Work out the finished part from the listing and answer in its coordinate system (mm). Face numbers are marked on the shaded views. A direction names the side the tool comes from. Give positions to 0.01 mm unless a question says otherwise; leave off trailing zeros. One line per item, written item: value.
from build123d import *

# Parameters (mm, degrees)
SKETCH1_W                   = 105
SKETCH1_H                   = 70
BOSS_EXTRUDE1_DEPTH         = 3
FILLET4_R                   = 3
FILLET5_R                   = 3
FILLET6_R                   = 3
M5X0_8_TAPPED_HOLE2_D       = 4.2
SKETCH16_6_W                = 34
SKETCH16_6_H                = 61
SKETCH16_6_W_2              = 30
SKETCH16_6_H_2              = 57
BOSS_EXTRUDE3_DEPTH         = 20
CUT_EXTRUDE8_REACH          = 129.334
SKETCH21_W                  = 30
SKETCH21_H                  = 57
SKETCH20_W                  = 34
SKETCH20_H                  = 61
BOSS_EXTRUDE4_DEPTH         = 2
SKETCH22_W                  = 34
SKETCH22_H                  = 61
CUT_EXTRUDE9_DEPTH          = 1.5
FILLET8_R                   = 3
SKETCH26_R                  = 6
CUT_EXTRUDE10_DEPTH         = 1.5
M3_TAPPED_HOLE1_D           = 2.5
M3_TAPPED_HOLE1_DEPTH       = 7.5
M3_TAPPED_HOLE1_TIP         = 0.751075774
SKETCH33_W                  = 1.5
SKETCH33_H                  = 5
CUT_EXTRUDE11_DEPTH         = 3
M3_TAPPED_HOLE2_D           = 2.5
M3_TAPPED_HOLE2_DEPTH       = 7.5
M3_TAPPED_HOLE2_TIP         = 0.751075774
M3_TAPPED_HOLE3_D           = 2.5
M3_TAPPED_HOLE3_DEPTH       = 7.5
M3_TAPPED_HOLE3_TIP         = 0.751075774
CUT_EXTRUDE12_REACH         = 101.423
SKETCH37_W                  = 10
SKETCH37_H                  = 10
SKETCH39_R                  = 3
CUT_EXTRUDE13_DEPTH         = 1.5
TAP_DRILL_FOR_M4X0_7_TAP2_D = 3.3


with BuildPart() as part:
    # Sketch1 → Boss-Extrude1 (new body)
    with BuildSketch(Plane.XY):
        with Locations((52.5, 35)):
            Rectangle(SKETCH1_W, SKETCH1_H)
    extrude(amount=BOSS_EXTRUDE1_DEPTH)

    # Fillet4
    fillet4_edges = [part.edges().sort_by_distance(p)[0] for p in [
        (105, 0, 1.5),
        (105, 70, 1.5),
    ]]
    fillet(fillet4_edges, radius=FILLET4_R)

    # Fillet5
    fillet5_edges = [part.edges().sort_by_distance(p)[0] for p in [
        (51, 70, 3),
        (105, 35, 3),
        (51, 0, 3),
        (104.121320344, 69.121320344, 3),
        (104.121320344, 0.878679656, 3),
    ]]
    fillet(fillet5_edges, radius=FILLET5_R - 0.0001)  # a hair under: the kernel refuses the full size

    # Fillet6
    fillet6_edges = [part.edges().sort_by_distance(p)[0] for p in [
        (0, 35, 3),
        (0, 0.878650367, 2.121349633),
        (0, 69.121349633, 2.121349633),
    ]]
    fillet(fillet6_edges, radius=FILLET6_R - 0.0001)  # a hair under: the kernel refuses the full size

    # M5x0.8 Tapped Hole2 (through all)
    with Locations(Plane(origin=(4, 66, 3), x_dir=(1, 0, 0), z_dir=(0, 0, 1))):
        with Locations((0, 0), (0, -62)):
            Hole(M5X0_8_TAPPED_HOLE2_D / 2)

    # Sketch16<6> → Boss-Extrude3 (add)
    with BuildSketch(Plane.XY.offset(3)):
        with Locations((83, 35)):
            Rectangle(SKETCH16_6_W, SKETCH16_6_H)
        with Locations((83, 35)):
            Rectangle(SKETCH16_6_W_2, SKETCH16_6_H_2, mode=Mode.SUBTRACT)
    extrude(amount=-BOSS_EXTRUDE3_DEPTH)

    # Sketch21 → Cut-Extrude8 (cut, up to next)
    with BuildSketch(Plane(origin=(0, 0, 0), x_dir=(-1, 0, 0), z_dir=(0, 0, -1)), mode=Mode.PRIVATE) as cut_extrude8_sk1:
        with Locations((-83, 35)):
            Rectangle(SKETCH21_W, SKETCH21_H)
    cut_extrude8_tool1 = extrude(cut_extrude8_sk1.sketch, amount=-CUT_EXTRUDE8_REACH, mode=Mode.PRIVATE) & part.part
    add(cut_extrude8_tool1.solids().sort_by_distance((83, 35, 0))[0], mode=Mode.SUBTRACT)

    # Sketch20 → Boss-Extrude4 (add)
    with BuildSketch(Plane(origin=(0, 0, -17), x_dir=(-1, 0, 0), z_dir=(0, 0, -1))):
        with Locations((-83, 35)):
            Rectangle(SKETCH20_W, SKETCH20_H)
    extrude(amount=BOSS_EXTRUDE4_DEPTH)

    # Sketch22 → Cut-Extrude9 (cut)
    with BuildSketch(Plane.XY.offset(3)):
        with Locations((83, 35)):
            Rectangle(SKETCH22_W, SKETCH22_H)
    extrude(amount=-CUT_EXTRUDE9_DEPTH, mode=Mode.SUBTRACT)

    # Fillet8
    fillet8_edges = [part.edges().sort_by_distance(p)[0] for p in [
        (100, 35, -19),
        (83, 4.5, -19),
        (66, 35, -19),
        (83, 65.5, -19),
    ]]
    fillet(fillet8_edges, radius=FILLET8_R)

    # Sketch26 → Cut-Extrude10 (cut)
    with BuildSketch(Plane.XY.offset(3)):
        with Locations((66, 35)):
            Circle(SKETCH26_R)
    extrude(amount=-CUT_EXTRUDE10_DEPTH, mode=Mode.SUBTRACT)

    # M3 Tapped Hole1
    with Locations(Plane(origin=(63, 35, 1.5), x_dir=(1, 0, 0), z_dir=(0, 0, 1))):
        with Locations((0, 0)):
            Hole(M3_TAPPED_HOLE1_D / 2, depth=M3_TAPPED_HOLE1_DEPTH)
            with Locations((0, 0, -(M3_TAPPED_HOLE1_DEPTH + M3_TAPPED_HOLE1_TIP / 2))):  # 118° drill point
                Cone(0, M3_TAPPED_HOLE1_D / 2, M3_TAPPED_HOLE1_TIP, mode=Mode.SUBTRACT)

    # Sketch33 → Cut-Extrude11 (cut)
    with BuildSketch(Plane.ZY.offset(-98)):
        with Locations((0.75, 51)):
            Rectangle(SKETCH33_W, SKETCH33_H)
        with Locations((0.75, 19)):
            Rectangle(SKETCH33_W, SKETCH33_H)
    extrude(amount=-CUT_EXTRUDE11_DEPTH, mode=Mode.SUBTRACT)

    # M3 Tapped Hole2
    with Locations(Plane(origin=(95.52684029, 8.597468083, -17), x_dir=(1, 0, 0), z_dir=(0, 0, 1))):
        with Locations((0, 0)):
            Hole(M3_TAPPED_HOLE2_D / 2, depth=M3_TAPPED_HOLE2_DEPTH)
            with Locations((0, 0, -(M3_TAPPED_HOLE2_DEPTH + M3_TAPPED_HOLE2_TIP / 2))):  # 118° drill point
                Cone(0, M3_TAPPED_HOLE2_D / 2, M3_TAPPED_HOLE2_TIP, mode=Mode.SUBTRACT)

    # M3 Tapped Hole3
    with Locations(Plane(origin=(95.52684029, 61.4, -17), x_dir=(1, 0, 0), z_dir=(0, 0, 1))):
        with Locations((0, 0)):
            Hole(M3_TAPPED_HOLE3_D / 2, depth=M3_TAPPED_HOLE3_DEPTH)
            with Locations((0, 0, -(M3_TAPPED_HOLE3_DEPTH + M3_TAPPED_HOLE3_TIP / 2))):  # 118° drill point
                Cone(0, M3_TAPPED_HOLE3_D / 2, M3_TAPPED_HOLE3_TIP, mode=Mode.SUBTRACT)

    # Sketch37 → Cut-Extrude12 (cut, up to next)
    with BuildSketch(Plane(origin=(68, 0, 0), x_dir=(0, 0, -1), z_dir=(1, 0, 0)), mode=Mode.PRIVATE) as cut_extrude12_sk1:
        with Locations((7.5, 53.5)):
            Rectangle(SKETCH37_W, SKETCH37_H)
    cut_extrude12_tool1 = extrude(cut_extrude12_sk1.sketch, amount=-CUT_EXTRUDE12_REACH, mode=Mode.PRIVATE) & part.part
    add(cut_extrude12_tool1.solids().sort_by_distance((68, 53.5, -7.5))[0], mode=Mode.SUBTRACT)

    # Sketch39 → Cut-Extrude13 (cut)
    with BuildSketch(Plane.XY.offset(3)):
        with Locations((60, 35)):
            Circle(SKETCH39_R)
    extrude(amount=-CUT_EXTRUDE13_DEPTH, mode=Mode.SUBTRACT)

    # Tap Drill for M4x0.7 Tap2 (through all)
    with Locations(Plane(origin=(20, 35, 3), x_dir=(1, 0, 0), z_dir=(0, 0, 1))):
        with Locations((0, 0), (15, 0)):
            Hole(TAP_DRILL_FOR_M4X0_7_TAP2_D / 2)


solid = part.part
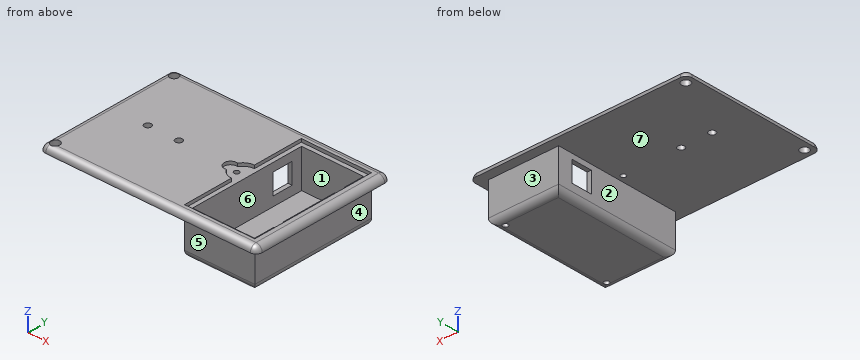
(1) Given P1, Ø2, axis at x = 98.5, y = 18.5, coming from the +Z side; P2, Ø12, axis at y = 51.5, z = -11, coming from the +X side; P3, Ø8, axis at x = 89, z = -9.5, coming from the +Y side, each flat-ended and moving along its own axis, determine where each tip first touches the part or whether it passes through.
Findings:
P1: stops at z = 0
P2: stops at x = 100
P3: stops at y = 65.5
(2) Which of the six approach directions +Z, -Z, +X, -X, +Y, -Y give full straight-line access (tool end or side, diameter ignored) to the marked faces 1, 2, 3 and 4?
Findings:
face 1: +Z
face 2: -Z, -X, +Y, -Y
face 3: -Z, +X, -X, +Y
face 4: -Z, +X, +Y, -Y
(3) Determine the mould class of the marked faces 5, 6 and 7 for opening direction Y: pulls with the +Y half, pulls with the -Y half, needs draft (parallel to the pull), parting line crosses it, or undercut.
Findings:
face 5: pulls with the -Y half
face 6: undercut
face 7: needs draft
(4) Find the intervals of material crossed by probe 1 along X at (y, z) = (51, -15.5); probe 2 along Y at (x, z) = (89, 0.25); probe 3 along Y at (x, z) = (94, -15.5), in increasing order. Write a range as from..to.
Findings:
probe 1: x = 66..68, 98..100
probe 2: y = 0.01..6.5, 63.5..69.99
probe 3: y = 4.5..6.5, 63.5..65.5
(5) Section B-B, the plane y = 35 is taken. Give the number of separate pieces and of enclosed holes in the cut face, then the cut area to 3 significant figures.
Findings:
separate pieces: 4
enclosed holes: 0
area: 310 mm^2
